Geometry check sheet. Reference: the model listing, model coordinates, mm. A direction names the side the tool comes from. Give positions to 0.01 mm unless a question says otherwise; leave off trailing zeros. Write each loop counter-clockwise with the first axis right and the second up, starting at its lowest first coordinate (ties: lowest second). Pieces come first, ordered by that corner, then holes.
(1) Cross-section at A-A (z = 0). Record the boundary of the cut face in (x, y), and give its area (3 significant figures).
(2) Cross-section at B-B (y = 0). Record the boundary of the cut face in (x, z).
(3) Cross-section at D-D (z = 7.75). Record the boundary of the cut face in (x, y).
(4) Cross-section at C-C (x = 2.05). Record the boundary of the cut face in (y, z), and give its area (3 significant figures).
(5) Depth check by flat-ended pin: P1, Ø1.5, axis at x = 1, z = -8.5, coming from the -Y side; P2, Ø0.9, axis at x = 1, y = -3, coming from the -Z side; P3, Ø4, axis at y = 0, z = 0, coming from the -X side; P4, Ø1.5, axis at x = 2, y = 2.5, coming from the +Z side. Enter the tip coordinate at first touch or a pass-through.
(6) Mould release check, pull along Y, two halves, no side actions. Record for faces 1 (the flat face through (1, 1.5, 9)), 2 (the cylindrical face through (1.48, 1.29, -0.17)), 3 (the flat face through (3, 2, 0)): +Y half, -Y half, draft (parallel to the pull), parting line (faces both ways), or undercut.
(7) Tool access check on faces 4 (the flat face through (1, 1.5, -9)), 5 (the flat face through (1, -3, 6)), 6 (the flat face through (1, -1.5, -9)), 7 (the flat face through (1, 3, 6)). Record the directions out of +Z, -Z, +X, -X, +Y, -Y that give a thin tool (end or side, any length) a straight path to the whole face; none if there is none.
(8) Thickness scan on line 1 along Y through (x, z) = (1.95, 0); line 2 along Z through (x, y) = (2.5, -2); line 3 along Z through (x, y) = (1.6, 1). Record the ranges inside material, lowest first.
```python
from build123d import *

# Parameters (mm, degrees)
PRINCIPAL_W                  = 12
PRINCIPAL_H                  = 3
PRINCIPAL_W_2                = 24
BASE_DEPTH                   = 3
FURO_DE_DI_METRO_2_6_2_6_1_D = 2.6


with BuildPart() as part:
    # Principal → Base (new body)
    with BuildSketch(Plane(origin=(0, 0, 0), x_dir=(0, 0, -1), z_dir=(1, 0, 0))):
        with Locations((0, 3)):
            Rectangle(PRINCIPAL_W, PRINCIPAL_H)
        Rectangle(PRINCIPAL_W_2, PRINCIPAL_H)
        with Locations((0, -3)):
            Rectangle(PRINCIPAL_W, PRINCIPAL_H)
    extrude(amount=BASE_DEPTH)

    # Furo de diâmetro Ø2.6 (2.6)1 (through all)
    with Locations(Plane(origin=(3, 0, 0), x_dir=(0, 0, -1), z_dir=(1, 0, 0))):
        with Locations((0, 0)):
            Hole(FURO_DE_DI_METRO_2_6_2_6_1_D / 2)


solid = part.part
```
Reply:
1. outline: (0, -4.5) - (3, -4.5) - (3, -1.3) - (0, -1.3) - close; (0, 1.3) - (3, 1.3) - (3, 4.5) - (0, 4.5) - close
1. area: 19.2 mm2
2. outline: (0, -12) - (3, -12) - (3, -1.3) - (0, -1.3) - close; (0, 1.3) - (3, 1.3) - (3, 12) - (0, 12) - close
3. outline: (0, -1.5) - (3, -1.5) - (3, 1.5) - (0, 1.5) - close
4. outline: (-4.5, -6) - (-1.5, -6) - (-1.5, -12) - (1.5, -12) - (1.5, -6) - (4.5, -6) - (4.5, 6) - (1.5, 6) - (1.5, 12) - (-1.5, 12) - (-1.5, 6) - (-4.5, 6) - close; hole circle Ø2.6 at (0, 0)
4. area: 139 mm2
5. P1: stops at y = -1.5
5. P2: stops at z = -6
5. P3: stops at x = 0
5. P4: stops at z = 6
6. face 1: +Y half
6. face 2: undercut
6. face 3: draft
7. face 4: -Z, +X, -X, +Y
7. face 5: +Z, +X, -X, -Y
7. face 6: -Z, +X, -X, -Y
7. face 7: +Z, +X, -X, +Y
8. line 1: y = -4.5 to -1.3, 1.3 to 4.5
8. line 2: z = -6 to 6
8. line 3: z = -12 to -0.83, 0.83 to 12
